Part model, mm, in its own coordinate system. A direction names the side the tool comes from. Give positions to 0.01 mm unless a question says otherwise; leave off trailing zeros. Write each loop counter-clockwise with the first axis right and the second up, starting at its lowest first coordinate (ties: lowest second). Pieces come first, ordered by that corner, then holes. Notation, with made-up numbers: (43, 14) - (54, 14) arc R21 ccw to (54, 42) - close; hole circle Ø2 at (75.5, 21). An arc over 180 degrees is marked (long way). Answer in a Markdown table with one row per item. Add a question column.
1. Which spindle directions (+Z, -Z, +X, -X, +Y, -Y) get a long thin tool onto all of the face, cutting with end or side? Do faces 1 (the flat face through (25, -35.35, 4)), 2 (the flat face through (-5.083, 2, 3)), 3 (the flat face through (-1.3, -32.4, 6)), 4 (the cylindrical face through (1.141, -26.497, 4.423)). Say none if no direction does.
2. Band-saw the part on A-A on x = 13.85. Write the cut outline in (y, z).
3. Pull direction X, two halves, no side cores. Call faces 5 (the cylindrical face through (23.412, 5.963, 5.415)), 6 (the flat face through (28, -14, -1)), 7 (the cylindrical face through (34.709, -34.147, 3.451)): released by +X, released by -X, zero draft, split by the parting line, or undercut.
4. Probe line 1 along X through (y, z) = (2, 0.25); line 2 along Y through (x, z) = (13.85, 11.15); line 3 along X through (y, z) = (-17.5, 3.5). List the from-to ranges inside material, lowest first.
5. Drop flat-ended pins along their axis: pin 1 Ø5 at (x, y) = (1, -24) entering from -Z; pin 2 Ø3.5 at (x, z) = (14.5, 3.5) entering from -Y; pin 3 Ø4 at (x, z) = (-2, 5.5) entering from -Y; pin 4 Ø2 at (x, z) = (31, 9) entering from -Y. Give the stop position or say it passes through.
6. Band-saw the part on C-C on y = -20.5. Write the cut outline in (x, z), plus the area to 3 significant figures.
7. Band-saw the part on B-B on z = 8.5. Write the cut outline in (x, y), plus the area to 3 significant figures.
8. Band-saw the part on D-D on y = -12.5. Write the cut outline in (x, z), plus the area to 3 significant figures.
```python
from build123d import *

# Parameters (mm, degrees)
SKETCH1_W                = 37.5
SKETCH1_H                = 40.9
SKETCH1_W_2              = 27.7
SKETCH1_H_2              = 27.7
BOSS_EXTRUDE1_DEPTH      = 6
SKETCH4_W                = 16.432066976
SKETCH4_H                = 47.432770651
CUT_EXTRUDE1_DEPTH       = 46
SKETCH5_W                = 44
SKETCH5_H                = 43
BOSS_EXTRUDE2_DEPTH      = 1
CUT_EXTRUDE2_DEPTH       = 1
SKETCH7_W                = 44
SKETCH7_H                = 43
SKETCH7_W_2              = 37.866148728
SKETCH7_H_2              = 40.8
BOSS_EXTRUDE3_DEPTH      = 6
FILLET1_R                = 4
SKETCH8_R                = 22
BOSS_EXTRUDE4_DEPTH      = 3
BOSS_EXTRUDE4_DEPTH_BACK = 8
SKETCH9_R                = 22
SKETCH9_R_2              = 18.5
BOSS_EXTRUDE5_DEPTH      = 3


with BuildPart() as part:
    # Sketch1 → Boss-Extrude1 (new body)
    with BuildSketch(Plane.XY):
        with Locations((13.85, -13.85)):
            Rectangle(SKETCH1_W, SKETCH1_H)
        with Locations((13.85, -13.85)):
            Rectangle(SKETCH1_W_2, SKETCH1_H_2, mode=Mode.SUBTRACT)
    extrude(amount=BOSS_EXTRUDE1_DEPTH)

    # Sketch4 → Cut-Extrude1 (cut)
    with BuildSketch(Plane.ZY.offset(4.9)):
        with Locations((3.592909633, -13.002986239)):
            Rectangle(SKETCH4_W, SKETCH4_H)
        with BuildLine():
            Line((0, 3.6), (0, -31.3))
            ThreePointArc((0, -31.3), (3, -34.3), (6, -31.3))
            Line((6, -31.3), (6, 3.6))
            ThreePointArc((6, 3.6), (3, 6.6), (0, 3.6))
        make_face(mode=Mode.SUBTRACT)
    extrude(amount=-CUT_EXTRUDE1_DEPTH, mode=Mode.SUBTRACT)

    # Sketch5 → Boss-Extrude2 (add)
    with BuildSketch(Plane.XY.offset(6)):
        with Locations((13.85, -13.85)):
            Rectangle(SKETCH5_W, SKETCH5_H)
    extrude(amount=BOSS_EXTRUDE2_DEPTH)

    # Sketch6 → Cut-Extrude2 (cut)
    with BuildSketch(Plane.XY.offset(7)):
        with BuildLine():
            Line((4, -27.7), (23.7, -27.7))
            ThreePointArc((23.7, -27.7), (26.528427125, -26.528427125), (27.7, -23.7))
            Line((27.7, -23.7), (27.7, -4))
            ThreePointArc((27.7, -4), (26.528427125, -1.171572875), (23.7, 0))
            Line((23.7, 0), (4, 0))
            ThreePointArc((4, 0), (1.171572875, -1.171572875), (0, -4))
            Line((0, -4), (0, -23.7))
            ThreePointArc((0, -23.7), (1.171572875, -26.528427125), (4, -27.7))
        make_face()
    extrude(amount=-CUT_EXTRUDE2_DEPTH, mode=Mode.SUBTRACT)

    # Sketch7 → Boss-Extrude3 (add)
    with BuildSketch(Plane(origin=(0, 0, 6), x_dir=(-1, 0, 0), z_dir=(0, 0, -1))):
        with Locations((-13.85, -13.85)):
            Rectangle(SKETCH7_W, SKETCH7_H)
        with Locations((-13.85, -13.85)):
            Rectangle(SKETCH7_W_2, SKETCH7_H_2, mode=Mode.SUBTRACT)
    extrude(amount=BOSS_EXTRUDE3_DEPTH)

    # Fillet1
    fillet1_edges = [part.edges().sort_by_distance(p)[0] for p in [
        (35.85, -35.35, 3.5),
        (35.85, 7.65, 3.5),
        (-8.15, 7.65, 3.5),
        (-8.15, -35.35, 3.5),
    ]]
    fillet(fillet1_edges, radius=FILLET1_R)

    # Sketch8 → Boss-Extrude4 (add, two sides)
    with BuildSketch(Plane.XY.offset(7)) as boss_extrude4_sk:
        with Locations((13.85, -13.85)):
            Circle(SKETCH8_R)
        with BuildLine():
            Line((27.7, -23.7), (27.7, -4))
            ThreePointArc((27.7, -4), (26.528427125, -1.171572875), (23.7, 0))
            Line((23.7, 0), (4, 0))
            ThreePointArc((4, 0), (1.171572875, -1.171572875), (0, -4))
            Line((0, -4), (0, -23.7))
            ThreePointArc((0, -23.7), (1.171572875, -26.528427125), (4, -27.7))
            Line((4, -27.7), (23.7, -27.7))
            ThreePointArc((23.7, -27.7), (26.528427125, -26.528427125), (27.7, -23.7))
        make_face(mode=Mode.SUBTRACT)
    extrude(amount=BOSS_EXTRUDE4_DEPTH)
    extrude(boss_extrude4_sk.sketch, amount=-BOSS_EXTRUDE4_DEPTH_BACK)

    # Sketch9 → Boss-Extrude5 (add)
    with BuildSketch(Plane.XY.offset(10)):
        with Locations((13.85, -13.85)):
            Circle(SKETCH9_R)
        with Locations((13.85, -13.85)):
            Circle(SKETCH9_R_2, mode=Mode.SUBTRACT)
    extrude(amount=BOSS_EXTRUDE5_DEPTH)


solid = part.part
```
Values:
| question | item | result |
|---|---|---|
| 1 | face 1 | +Z, -Z, +X, -Y |
| 1 | face 2 | -Z |
| 1 | face 3 | none |
| 1 | face 4 | +Z, -Z |
| 2 | outline | (-35.85, -1) - (-27.7, -1) - (-27.7, 10) - (-32.35, 10) - (-32.35, 13) - (-35.85, 13) - close; (0, -1) - (8.15, -1) - (8.15, 13) - (4.65, 13) - (4.65, 10) - (0, 10) - close |
| 3 | face 5 | undercut |
| 3 | face 6 | zero draft |
| 3 | face 7 | released by +X |
| 4 | line 1 | x = -8.15 to -5.08, -4.9 to 32.6, 32.78 to 35.85 |
| 4 | line 2 | y = -35.85 to -32.35, 4.65 to 8.15 |
| 4 | line 3 | x = -8.15 to 0, 27.7 to 35.85 |
| 5 | pin 1 | stops at z = -1 |
| 5 | pin 2 | stops at y = -35.85 |
| 5 | pin 3 | stops at y = -35.35 |
| 5 | pin 4 | stops at y = -28.79 |
| 6 | outline | (-8.15, 0) - (-7.12, 0) - (-7.12, -1) - (0, -1) - (0, 10) - (-3.41, 10) - (-3.41, 13) - (-7.12, 13) - (-7.12, 7) - (-8.15, 7) - close; (27.7, -1) - (34.82, -1) - (34.82, 0) - (35.85, 0) - (35.85, 7) - (34.82, 7) - (34.82, 13) - (31.11, 13) - (31.11, 10) - (27.7, 10) - close |
| 6 | area | 193 mm² |
| 7 | outline | circle Ø44 at (13.85, -13.85); hole (0, -23.7) arc R4 ccw to (4, -27.7) - (23.7, -27.7) arc R4 ccw to (27.7, -23.7) - (27.7, -4) arc R4 ccw to (23.7, 0) - (4, 0) arc R4 ccw to (0, -4) - close |
| 7 | area | 767 mm² |
| 8 | outline | (-8.15, 0) - (-8.11, 0) - (-8.11, -1) - (0, -1) - (0, 10) - (-4.6, 10) - (-4.6, 13) - (-8.11, 13) - (-8.11, 7) - (-8.15, 7) - close; (27.7, -1) - (35.81, -1) - (35.81, 0) - (35.85, 0) - (35.85, 7) - (35.81, 7) - (35.81, 13) - (32.3, 13) - (32.3, 10) - (27.7, 10) - close |
| 8 | area | 200 mm² |
